Job drawing, mm, ordinate dimensions from the low corner. One solid piece. A direction names the side the tool comes from. Round coordinates to 2 decimals unless told otherwise and drop trailing zeros. Write each loop counter-clockwise with the first axis right and the second up, starting at its lowest first coordinate (ties: lowest second). Pieces come first, ordered by that corner, then holes. Notation, with made-up numbers: M 47.25,4 L 54.25,4 A17 cw 54.25,33 Z; hole C 31,-29.75 d7. An arc over 180 degrees is marked long. Write each question's results on one line, items separated by ' | '. Start each with the question number.
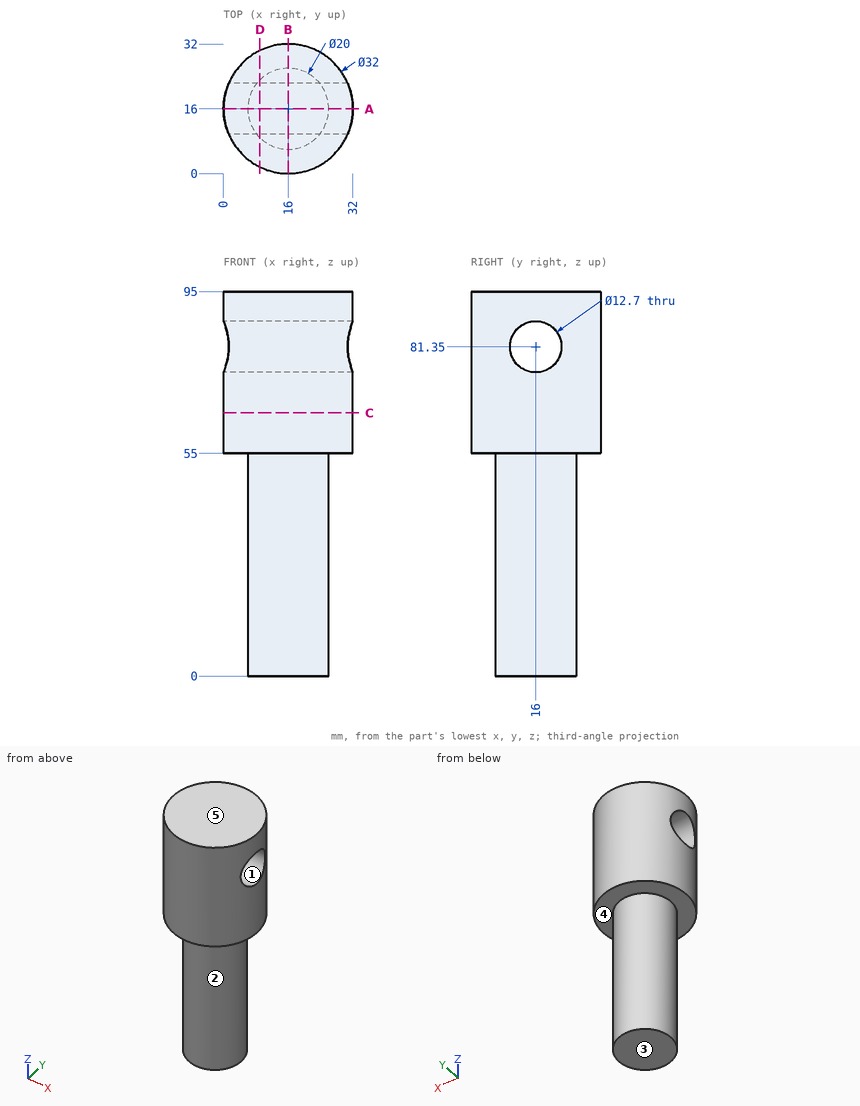
1) Drop flat-ended pins along their axis: pin 1 Ø10 at (y, z) = (26.5, 49) entering from +X; pin 2 Ø12 at (y, z) = (4, 76.5) entering from -X; pin 3 Ø4 at (y, z) = (13.5, 44) entering from +X. Give the stop position or say it passes through.
2) Wall check: line 1 along Z through (x, y) = (26.5, 4); line 2 along Y through (x, z) = (16, 81); line 3 along Y through (x, z) = (14, 81.35). Give the ranges that are in metal, low to high. Write a range as from..to.
3) Saw through at C-C, the plane z = 65. Write the cut outline in (x, y), plus the area to 3 significant figures.
4) Saw through at A-A, the plane y = 16. Write the cut outline in (x, z).
5) Saw through at B-B, the plane x = 16. Write the cut outline in (y, z).
6) 3-axis set-ups, long thin cutter, end or side, ignore diameter. For the marked faces 4 and 5: which of +Z, -Z, +X, -X, +Y, -Y reach the whole face in a straight line?
7) Pull direction Y, two halves, no side cores. Call the marked faces 1, 2 and 3: pulls with the +Y half, pulls with the -Y half, needs draft (parallel to the pull), parting line crosses it, or undercut.
8) Saw through at D-D, the plane x = 9. Write the cut outline in (y, z), plus the area to 3 significant figures.
Filled sheet:
1) pin 1: stops at x = 24.35 | pin 2: stops at x = 1.17 | pin 3: stops at x = 25.99
2) line 1: z = 55..95 | line 2: y = 0..9.66, 22.34..32 | line 3: y = 0.13..9.65, 22.35..31.87
3) outline: C 16,16 d32 | area: 804 mm^2
4) outline: M 0,55 L 6,55 L 6,0 L 26,0 L 26,55 L 32,55 L 32,75 L 0,75 Z; M 0,87.7 L 32,87.7 L 32,95 L 0,95 Z
5) outline: M 0,55 L 6,55 L 6,0 L 26,0 L 26,55 L 32,55 L 32,95 L 0,95 Z; hole C 16,81.35 d12.7
6) face 4: -Z | face 5: +Z, +X, -X, +Y, -Y
7) face 1: undercut | face 2: parting line crosses it | face 3: needs draft
8) outline: M 1.61,55 L 8.86,55 L 8.86,0 L 23.14,0 L 23.14,55 L 30.39,55 L 30.39,95 L 1.61,95 Z; hole C 16,81.35 d12.7 | area: 1,810 mm^2
